from build123d import *

# Parameters (mm, degrees)
F0_W            = 84
F0_H            = 84
F1_DEPTH        = 10
F2_W            = 80
F2_H            = 80
F3_DEPTH        = 9.5
F4_W            = 84
F4_H            = 84
F5_DEPTH        = 10
F6_SIZE2        = 9.99999
F6_SIZE         = 41.99999
F8_D            = 3.4
F8_DEPTH        = 12
F8_CSINK_D      = 6.72
F8_CSINK_ANGLE  = 90
F8_TIP          = 1.0214630523
F10_D           = 3.4
F10_DEPTH       = 12
F10_CSINK_D     = 6.72
F10_CSINK_ANGLE = 90
F10_TIP         = 1.0214630523


# Not quite as in the source:
# - a fillet or chamfer is up to 0.001 mm smaller than in the source, because OpenCascade refuses the exact size


with BuildPart() as f1:
    # F0 (on Top) → F1 (new body)
    with BuildSketch(Plane.XY):
        with Locations((42, 42)):
            Rectangle(F0_W, F0_H)
    extrude(amount=F1_DEPTH)

    # F2 (on face) → F3 (cut)
    with BuildSketch(Plane(origin=(0, 0, 0), x_dir=(1, 0, 0), z_dir=(0, 0, -1))):
        with Locations((42, -42)):
            Rectangle(F2_W, F2_H)
    extrude(amount=-F3_DEPTH, mode=Mode.SUBTRACT)

    # F4 (on face) → F5 (join)
    with BuildSketch(Plane.XY.offset(10)):
        with Locations((42, 42)):
            Rectangle(F4_W, F4_H)
    extrude(amount=F5_DEPTH)

    # F6 (size 42 and 10 in the source; OpenCascade refuses exactly that, so slightly less here)
    f6_edges = [f1.edges().sort_by_distance(p)[0] for p in [
        (0, 42, 20),
        (42, 84, 20),
        (84, 42, 20),
        (42, 0, 20),
    ]]
    f6_side = f1.faces().sort_by_distance((42, 42, 20))[0]
    chamfer(f6_edges, length=F6_SIZE, length2=F6_SIZE2, reference=f6_side)

    # F8
    with Locations(Plane.XZ):
        with Locations((42, 5)):
            CounterSinkHole(F8_D / 2, F8_CSINK_D / 2, depth=F8_DEPTH, counter_sink_angle=F8_CSINK_ANGLE)
            with Locations((0, 0, -(F8_DEPTH + F8_TIP / 2))):  # 118° drill point
                Cone(0, F8_D / 2, F8_TIP, mode=Mode.SUBTRACT)

    # F10
    with Locations(Plane(origin=(0, 84, 0), x_dir=(-1, 0, 0), z_dir=(0, 1, 0))):
        with Locations((-42, 5)):
            CounterSinkHole(F10_D / 2, F10_CSINK_D / 2, depth=F10_DEPTH, counter_sink_angle=F10_CSINK_ANGLE)
            with Locations((0, 0, -(F10_DEPTH + F10_TIP / 2))):  # 118° drill point
                Cone(0, F10_D / 2, F10_TIP, mode=Mode.SUBTRACT)


solid = f1.part
Here's how the part is built. I have some questions about the finished solid (model axes, mm). A direction names the side the tool comes from. Coordinates: 2 decimals unless noted, no trailing zeros. Write each loop counter-clockwise with the first axis right and the second up, starting at its lowest first coordinate (ties: lowest second). Pieces come first, ordered by that corner, then holes. Notation, with made-up numbers: (-13, 63.25) - (26, 63.25) arc R21 cw to (26, 81.25) - close; hole circle Ø10 at (-27, -11). An arc over 180 degrees is marked (long way). Use one line per item in the form item = value.
1) I'm going to push flat-ended pins straight in: P1, Ø4, axis at x = 42, z = 5, coming from the -Y side; P2, Ø8, axis at x = 73.5, y = 31.5, coming from the -Z side; P3, Ø3, axis at x = 64, y = 34, coming from the +Z side. Where does each tip first touch, or does it pass through?
Solved:
P1 = 1.36
P2 = 9.5
P3 = 15.12
2) Suppose I cut it at C-C, the plane y = 14.5. Write out the boundary of the cut face in (x, z), plus the area to 3 significant figures.
Solved:
outline = (0, 0) - (2, 0) - (2, 9.5) - (82, 9.5) - (82, 0) - (84, 0) - (84, 10) - (69.5, 13.45) - (14.5, 13.45) - (0, 10) - close
area = 320 mm2
3) Thinking about a two-plate mould opening in X: for faces 1 (the cylindrical face through (43.35, 1.83, 3.97)), 2 (the flat face through (41.4, 0, 0.5)), 3 (the flat face through (84, 41, 5)), which applies, released by +X, released by -X, zero draft, split by the parting line, or undercut?
Solved:
face_1 = undercut
face_2 = zero draft
face_3 = released by +X
4) Suppose I cut it at A-A, the plane z = 5. Write out the boundary of the cut face in (x, y), plus the area to 3 significant figures.
Solved:
outline = (0, 0) - (38.64, 0) - (40.3, 1.66) - (40.3, 2) - (2, 2) - (2, 82) - (40.3, 82) - (40.3, 82.34) - (38.64, 84) - (0, 84) - close; (43.7, 1.66) - (45.36, 0) - (84, 0) - (84, 84) - (45.36, 84) - (43.7, 82.34) - (43.7, 82) - (82, 82) - (82, 2) - (43.7, 2) - close
area = 637 mm2
5) I need wall thicknesses on line 1 (X direction, y = 1.8, z = 5); line 2 (X direction, y = 12, z = 3.5). Which ranges of each line are inside material? Lowest first, please.
Solved:
line_1 = 0 to 40.3, 43.7 to 84
line_2 = 0 to 2, 82 to 84
6) Suppose I cut it at D-D, the plane z = 14. Write out the boundary of the cut face in (x, y), plus the area to 3 significant figures.
Solved:
outline = (16.8, 16.8) - (67.2, 16.8) - (67.2, 67.2) - (16.8, 67.2) - close
area = 2,540 mm2
7) On a 3-axis mill with a long thin cutter (end or side, diameter ignored), from which of +Z, -Z, +X, -X, +Y, -Y can I reach the whole of each face in a straight line? I mean faces 4 (the flat face through (16.04, 41.41, 13.82)), 5 (the flat face through (2, 43, 5)). Say none if no direction works.
Solved:
face_4 = +Z, -X, +Y, -Y
face_5 = -Z
8) Suppose I cut it at B-B, the plane x = 30. Write out the boundary of the cut face in (y, z), plus the area to 3 significant figures.
Solved:
outline = (0, 0) - (2, 0) - (2, 9.5) - (82, 9.5) - (82, 0) - (84, 0) - (84, 10) - (54, 17.14) - (30, 17.14) - (0, 10) - close
area = 466 mm2
